Could you check a few things on this model? Use its own coordinates, in mm. Face numbers are marked on the shaded views. Round coordinates to 2 decimals unless told otherwise and drop trailing zeros. Order: outer loops, then holes, each group sorted by start corner. A loop starts at its lowest first (then second) coordinate and runs counter-clockwise, first axis right, second up. Notation, with made-up numbers: (58.5, -23.5) -> (65.5, -23.5) arc R28 cw to (65.5, 14.5) -> close; hole circle Ø10 at (68.5, -29.75). An arc over 180 degrees is marked (long way). One line per question, with ' | ' between items.
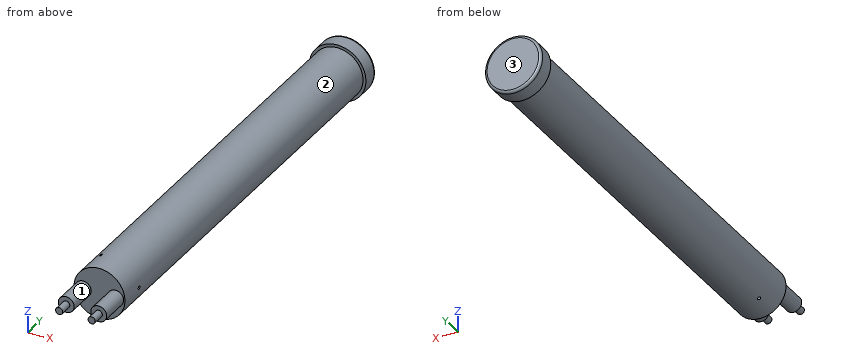
```python
from build123d import *

# Parameters (mm, degrees)
SKETCH1_R                = 20
BOSS_EXTRUDE1_DEPTH      = 345
BOSS_EXTRUDE2_DEPTH      = 5
BOSS_EXTRUDE2_DEPTH_BACK = 8.5
SKETCH2_R                = 22.25
FILLET1_R                = 2
SKETCH3_R                = 1.25
CUT_EXTRUDE1_DEPTH       = 5
CIRPATTERN1_COUNT        = 3
SKETCH4_R                = 6.25
BOSS_EXTRUDE3_DEPTH      = 24
SKETCH5_R                = 2.8
BOSS_EXTRUDE4_DEPTH      = 10


with BuildPart() as part:
    # Sketch1 → Boss-Extrude1 (new body)
    with BuildSketch(Plane(origin=(0, 0, 0), x_dir=(1, 0, 0), z_dir=(0, 1, 0))):
        with Locations(Location((0, 0, 0), (0, 0, 270))):
            Circle(SKETCH1_R)
    extrude(amount=BOSS_EXTRUDE1_DEPTH)

    # Sketch2 → Boss-Extrude2 (add, two sides: drawn at the far end of the back side and taken through both)
    with BuildSketch(Plane(origin=(0, 345, 0), x_dir=(1, 0, 0), z_dir=(0, 1, 0)).offset(-BOSS_EXTRUDE2_DEPTH_BACK)):
        with Locations(Location((0, 0, 0), (0, 0, 270))):
            Circle(SKETCH2_R)
    extrude(amount=BOSS_EXTRUDE2_DEPTH + BOSS_EXTRUDE2_DEPTH_BACK)

    # Fillet1
    fillet1_edges = [part.edges().sort_by_distance(p)[0] for p in [
        (0, 350, -22.25),
    ]]
    fillet(fillet1_edges, radius=FILLET1_R)

    # Sketch3 → Cut-Extrude1 (cut)
    with BuildSketch(Plane(origin=(20, 0, 0), x_dir=(0, 0, -1), z_dir=(1, 0, 0))):
        with Locations((0, 20)):
            Circle(SKETCH3_R)
    cut_extrude1 = extrude(amount=-CUT_EXTRUDE1_DEPTH, mode=Mode.SUBTRACT)

    # CirPattern1: Cut-Extrude1 ×3 about axis
    cirpattern1_axis = Axis((0, 0, 0), (0, 1, 0))
    for i in range(1, CIRPATTERN1_COUNT):
        add(cut_extrude1.rotate(cirpattern1_axis, i * 360 / CIRPATTERN1_COUNT), mode=Mode.SUBTRACT)

    # Sketch4 → Boss-Extrude3 (add)
    with BuildSketch(Plane.XZ):
        with Locations(Location((-12.75, 0, 0), (0, 0, 90))):
            Circle(SKETCH4_R)
        with Locations(Location((12.75, 0, 0), (0, 0, 90))):
            Circle(SKETCH4_R)
    extrude(amount=BOSS_EXTRUDE3_DEPTH)

    # Sketch5 → Boss-Extrude4 (add)
    with BuildSketch(Plane.XZ.offset(24)):
        with Locations(Location((-12.75, 0, 0), (0, 0, 270))):
            Circle(SKETCH5_R)
        with Locations(Location((12.75, 0, 0), (0, 0, 270))):
            Circle(SKETCH5_R)
    extrude(amount=BOSS_EXTRUDE4_DEPTH)


solid = part.part
```
1. I want a section at A-A on x = 0. List the corners of the cut face in (y, z) for me.
From the geometry:
outline: (0, -20) -> (336.5, -20) -> (336.5, -22.25) -> (348, -22.25) arc R2 ccw to (350, -20.25) -> (350, 20.25) arc R2 ccw to (348, 22.25) -> (336.5, 22.25) -> (336.5, 20) -> (0, 20) -> close
2. I'm going to push flat-ended pins straight in: pin 1 (8 mm diameter, centred on x = -5, y = 302.5, fed in from +Z) (3 decimals); pin 2 (1 mm diameter, centred on x = 18, z = 3, fed in from -Y); pin 3 (12 mm diameter, centred on x = -14.5, y = 61, fed in from -Z). Where does each tip first touch, or does it pass through?
From the geometry:
pin 1: stops at z = 19.975 | pin 2: stops at y = -24 | pin 3: stops at z = -18.1
3. I want a section at C-C on y = -4.5. List the corners of the cut face in (x, z) for me.
From the geometry:
outline: circle Ø12.5 at (-12.75, 0); circle Ø12.5 at (12.75, 0)
4. I need wall thicknesses on probe 1 along Y at (x, z) = (17, 0); probe 2 along X at (y, z) = (27, 6); probe 3 along Y at (x, z) = (-8, 0.5). Which ranges of each line are inside material? Lowest first, please.
From the geometry:
probe 1: y = -24 to 18.75, 21.25 to 350 | probe 2: x = -19.08 to 19.08 | probe 3: y = -24 to 350
5. If we mould it in two halves opening along X, with no side actions, what happens to the marked faces 1, 2 and 3? For each: pulls with the +X half, pulls with the -X half, needs draft (parallel to the pull), parting line crosses it, or undercut.
From the geometry:
face 1: undercut | face 2: parting line crosses it | face 3: needs draft
6. I want a section at B-B on y = 273. List the corners of the cut face in (x, z) for me, and give its area (3 significant figures).
From the geometry:
outline: circle Ø40 at (0, 0) | area: 1,260 mm²
